from build123d import *

# Parameters (mm, degrees)
SKETCH4_W            = 127
SKETCH4_H            = 83
BOSS_EXTRUDE3_DEPTH  = 30
SKETCH10_R           = 9.5
CUT_EXTRUDE11_DEPTH  = 80.871772235
SKETCH8_R            = 2.5
CUT_EXTRUDE9_DEPTH   = 3.7
SKETCH8_11_R         = 2.2352
CUT_EXTRUDE10_DEPTH  = 82.575118756
CUT_EXTRUDE12_START  = -82.575118756
SKETCH8_12_R         = 4.0132
SKETCH8_12_R_2       = 2.2352
CUT_EXTRUDE12_DEPTH  = 83.641918756
LPATTERN4_COUNT      = 6
LPATTERN4_PITCH      = 20
LPATTERN4_COUNT_DIR2 = 4
LPATTERN4_PITCH_DIR2 = 20
SKETCH8_13_R         = 6.4008
SKETCH8_13_R_2       = 4.6228
CUT_EXTRUDE16_DEPTH  = 1.3208
LPATTERN5_COUNT      = 5
LPATTERN5_PITCH      = 20
LPATTERN5_COUNT_DIR2 = 3
LPATTERN5_PITCH_DIR2 = 20


with BuildPart() as part:
    # Sketch4 → Boss-Extrude3 (new body)
    with BuildSketch(Plane(origin=(0, 10, 0), x_dir=(1, 0, 0), z_dir=(0, 1, 0))):
        Rectangle(SKETCH4_W, SKETCH4_H)
    extrude(amount=BOSS_EXTRUDE3_DEPTH)

    # Sketch10 → Cut-Extrude11 (cut, through all)
    with BuildSketch(Plane(origin=(0, 15, 0), x_dir=(1, 0, 0), z_dir=(0, 1, 0))):
        with Locations(Location((-40.08, -20, 0), (0, 0, 270))):
            Circle(SKETCH10_R)
    cut_extrude11 = extrude(amount=CUT_EXTRUDE11_DEPTH, mode=Mode.SUBTRACT)

    # Sketch8 → Cut-Extrude9 (cut)
    with BuildSketch(Plane(origin=(0, 10, 0), x_dir=(1, 0, 0), z_dir=(0, 1, 0))):
        with Locations(Location((-50.08, -30, 0), (0, 0, 270))):
            Circle(SKETCH8_R)
    cut_extrude9 = extrude(amount=CUT_EXTRUDE9_DEPTH, mode=Mode.SUBTRACT)

    # Sketch8_11 → Cut-Extrude10 (cut, through all)
    with BuildSketch(Plane(origin=(0, 10, 0), x_dir=(1, 0, 0), z_dir=(0, 1, 0))):
        with Locations(Location((-40.08, -20, 0), (0, 0, 270))):
            Circle(SKETCH8_11_R)
    cut_extrude10 = extrude(amount=CUT_EXTRUDE10_DEPTH, mode=Mode.SUBTRACT)

    # Sketch8_12 → Cut-Extrude12 (cut)
    with BuildSketch(Plane(origin=(0, 10, 0), x_dir=(1, 0, 0), z_dir=(0, 1, 0)).offset(CUT_EXTRUDE12_START)):
        with Locations(Location((-40.08, -20, 0), (0, 0, 270))):
            Circle(SKETCH8_12_R)
        with Locations(Location((-40.08, -20, 0), (0, 0, 270))):
            Circle(SKETCH8_12_R_2, mode=Mode.SUBTRACT)
    cut_extrude12 = extrude(amount=CUT_EXTRUDE12_DEPTH, mode=Mode.SUBTRACT)

    # LPattern4: Cut-Extrude9 6 × 4
    with Locations(*[(i * LPATTERN4_PITCH, 0, -j * LPATTERN4_PITCH_DIR2) for i in range(LPATTERN4_COUNT) for j in range(LPATTERN4_COUNT_DIR2) if (i, j) != (0, 0)]):
        add(cut_extrude9, mode=Mode.SUBTRACT)

    # Sketch8_13 → Cut-Extrude16 (cut)
    with BuildSketch(Plane(origin=(0, 10, 0), x_dir=(1, 0, 0), z_dir=(0, 1, 0))):
        with Locations(Location((-40.08, -20, 0), (0, 0, 270))):
            Circle(SKETCH8_13_R)
        with Locations(Location((-40.08, -20, 0), (0, 0, 270))):
            Circle(SKETCH8_13_R_2, mode=Mode.SUBTRACT)
    cut_extrude16 = extrude(amount=CUT_EXTRUDE16_DEPTH, mode=Mode.SUBTRACT)

    # LPattern5: Cut-Extrude11, Cut-Extrude10, Cut-Extrude12, Cut-Extrude16 5 × 3
    with Locations(*[(i * LPATTERN5_PITCH, 0, -j * LPATTERN5_PITCH_DIR2) for i in range(LPATTERN5_COUNT) for j in range(LPATTERN5_COUNT_DIR2) if (i, j) != (0, 0)]):
        add(cut_extrude11, mode=Mode.SUBTRACT)
        add(cut_extrude10, mode=Mode.SUBTRACT)
        add(cut_extrude12, mode=Mode.SUBTRACT)
        add(cut_extrude16, mode=Mode.SUBTRACT)


solid = part.part
Can you work these out from the model? Positions are in its coordinate system, mm. A direction names the side the tool comes from. Coordinates: 2 decimals unless noted, no trailing zeros. Write each question's results on one line, items separated by ' | '. Start each with the question number.
Q1. If I drill on probe 1 along X at (y, z) = (30, 0); probe 2 along Z at (x, y) = (19.92, 20.25); probe 3 along Z at (x, y) = (-49, 11.75), over which ranges is the centre line in solid material (lowest first)?
Q2. We'd pull the mould along X, two halves only. Please class faces 1 (the face through (36, 10, 18)), 2 (the face through (10, 13.7, 10)): +X half, -X half, draft (parallel to the pull), parting line (faces both ways), or undercut.
Q3. On a 3-axis mill with a long thin cutter (end or side, diameter ignored), from which of +Z, -Z, +X, -X, +Y, -Y can I reach the whole of each face in a straight line? I mean faces 3 (the face through (50, 13.7, 30)), 4 (the face through (-37.864, 13.006, -20.291)), 5 (the face through (-42, 15, -18)). Say none if no direction works.
Q4. I'm going to push flat-ended pins straight in: pin 1 (4 mm diameter, centred on x = 19.5, z = 0, fed in from +Y); pin 2 (1.5 mm diameter, centred on x = 10, z = 29.5, fed in from -Y). Where does each tip first touch, or does it pass through?
Q5. Imagine slicing it at A-A (y = 38). State how many separate pieces and enclosed holes the cut face has, then the cut area to 3 significant figures.
Taken from the geometry:
1) probe 1: x = -63.5 to -49.58, -30.58 to -29.58, -10.58 to -9.58, 9.42 to 10.42, 29.42 to 30.42, 49.42 to 63.5 | probe 2: z = -41.5 to -29.5, -10.5 to -9.5, 9.5 to 10.5, 29.5 to 41.5 | probe 3: z = -41.5 to -32.25, -27.75 to -12.25, -7.75 to 7.75, 12.25 to 27.75, 32.25 to 41.5
2) face 1: draft | face 2: undercut
3) face 3: -Y | face 4: +Y, -Y | face 5: +Y
4) pin 1: stops at y = 15 | pin 2: stops at y = 13.7
5) separate pieces: 1 | enclosed holes: 15 | area: 6,290 mm^2
